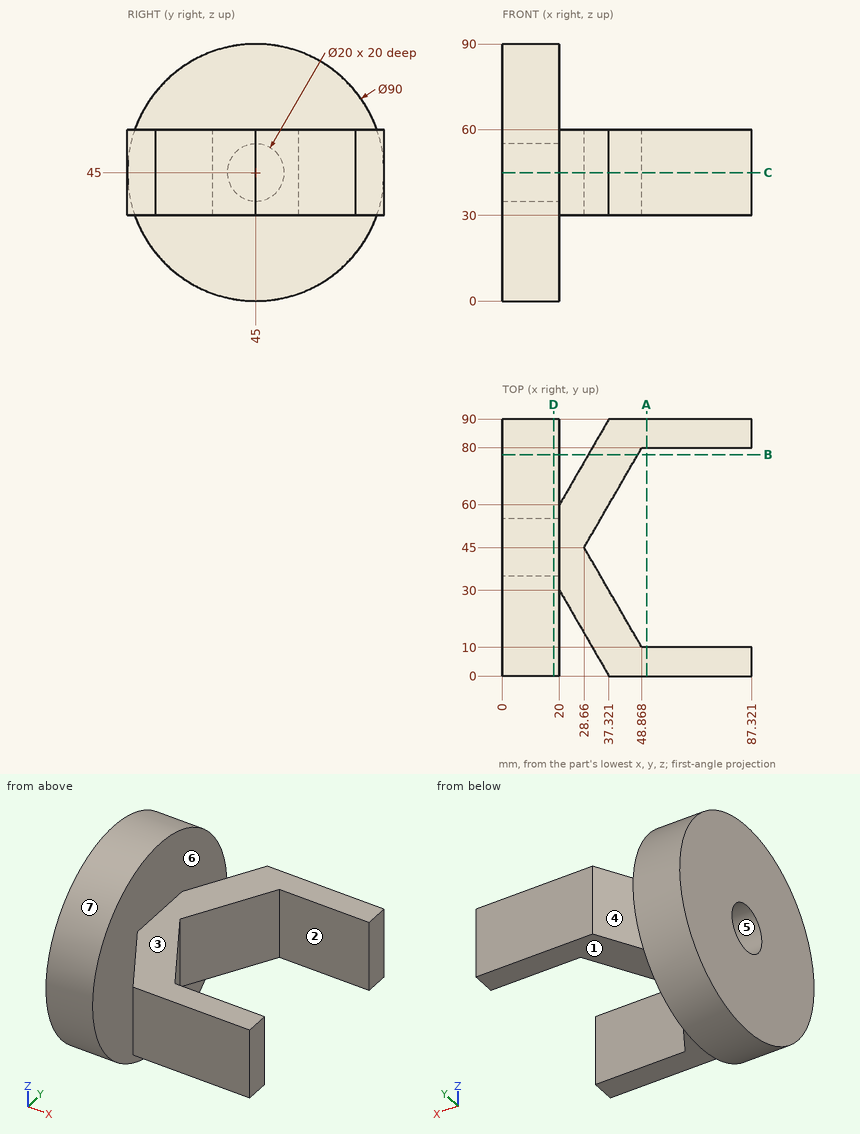
Here's the drawing with two shaded views (mm, measured from the low corner). I have some questions. A direction names the side the tool comes from. Give positions to 0.01 mm unless a question says otherwise; leave off trailing zeros. Order: outer loops, then holes, each group sorted by start corner. A loop starts at its lowest first (then second) coordinate and runs counter-clockwise, first axis right, second up.
Q1. Suppose I cut it at A-A, the plane x = 50.5. Write out the boundary of the cut face in (y, z), and give its area (3 significant figures).
Q2. I'm going to push flat-ended pins straight in: P1, Ø10, axis at x = 16, z = 20.5, coming from the +Y side (1 decimal); P2, Ø2, axis at y = 49, z = 38, coming from the +X side; P3, Ø1.5, axis at x = 38.5, y = 66, coming from the -Z side; P4, Ø1, axis at x = 69, z = 58, coming from the -Y side. Where does each tip first touch, or does it pass through?
Q3. Suppose I cut it at C-C, the plane z = 45. Write out the boundary of the cut face in (x, y), and give its area (3 significant figures).
Q4. We'd pull the mould along Y, two halves only. Please class the marked faces 4, 5, 6 and 7: +Y half, -Y half, draft (parallel to the pull), parting line (faces both ways), or undercut.
Q5. Suppose I cut it at D-D, the plane x = 18. Write out the boundary of the cut face in (y, z), and give its area (3 significant figures).
Q6. If I drill on line 1 along Y through (x, z) = (10, 45); line 2 along Y through (x, z) = (55, 38.5); line 3 along X through (y, z) = (42.5, 14), over which ranges is the centre line in solid material (lowest first)?
Q7. For the marked faces 1, 2 and 3, which set-ups out of +Z, -Z, +X, -X, +Y, -Y let a thin tool reach every point of the face, with its end or its side?
Q8. Suppose I cut it at B-B, the plane y = 77.5. Write out the boundary of the cut face in (x, z) (1 decimal).
Solution:
1. outline: (0, 30) - (10, 30) - (10, 60) - (0, 60) - close; (80, 30) - (90, 30) - (90, 60) - (80, 60) - close
1. area: 600 mm2
2. P1: stops at y = 85.6
2. P2: stops at x = 31.55
2. P3: stops at z = 30
2. P4: stops at y = 0
3. outline: (0, 0) - (20, 0) - (20, 30) - (37.32, 0) - (87.32, 0) - (87.32, 10) - (48.87, 10) - (28.66, 45) - (48.87, 80) - (87.32, 80) - (87.32, 90) - (37.32, 90) - (20, 60) - (20, 90) - (0, 90) - (0, 55) - (20, 55) - (20, 35) - (0, 35) - close
3. area: 3,540 mm2
4. face 4: +Y half
4. face 5: undercut
4. face 6: draft
4. face 7: parting line
5. outline: circle Ø90 at (45, 45); hole circle Ø20 at (45, 45)
5. area: 6,050 mm2
6. line 1: y = 0 to 35, 55 to 90
6. line 2: y = 0 to 10, 80 to 90
6. line 3: x = 0 to 20
7. face 1: -Z, +X, +Y, -Y
7. face 2: +Z, -Z, +X
7. face 3: +Z, +X, +Y, -Y
8. outline: (0, 13.9) - (20, 13.9) - (20, 76.1) - (0, 76.1) - close; (30.1, 30) - (47.4, 30) - (47.4, 60) - (30.1, 60) - close
